Design review of the part shown in the three views and the two pictorial views. Dimensions are in mm from the part's minimum x, y and z. Give positions to 0.01 mm unless a question says otherwise; leave off trailing zeros. Order: outer loops, then holes, each group sorted by start corner. A loop starts at its lowest first (then second) coordinate and runs counter-clockwise, first axis right, second up. Notation, with made-up numbers: (-13, 73.25) - (20, 73.25) arc R17 cw to (20, 106.25) - close; hole circle Ø7 at (-23.5, 78). An arc over 180 degrees is marked (long way). Put each result on its own line as item: value.
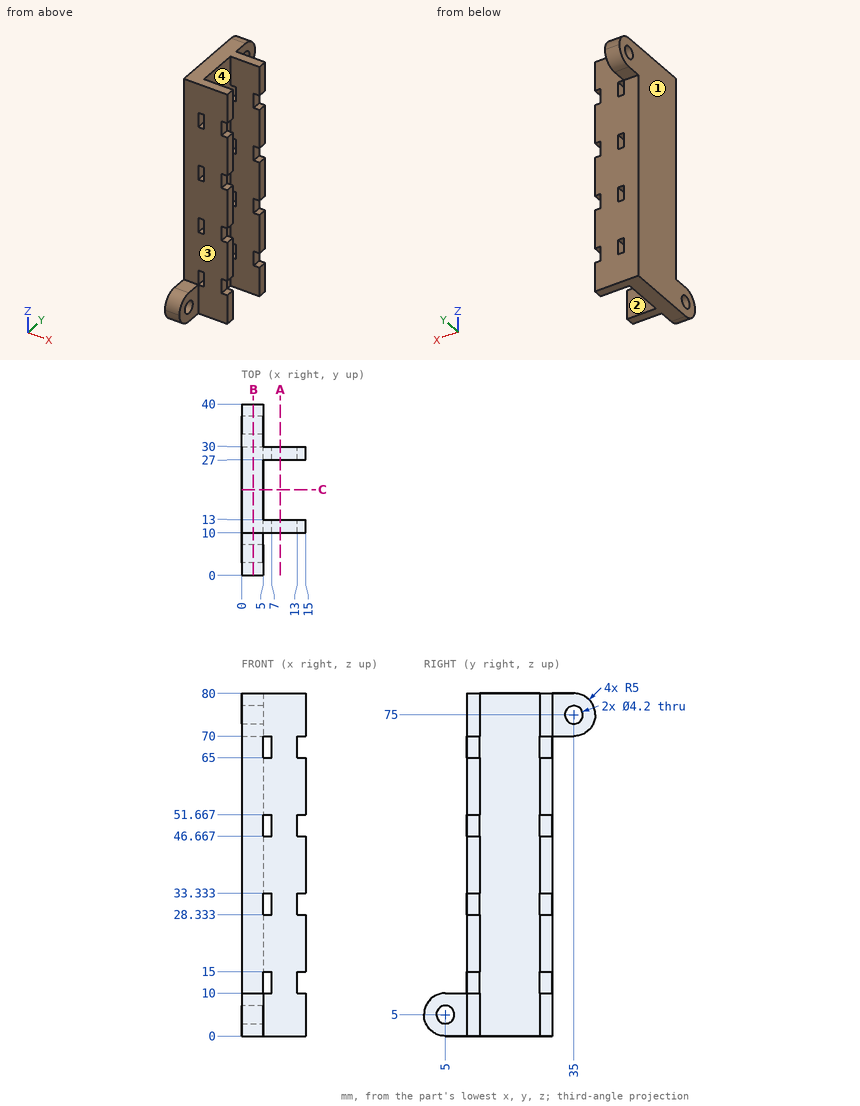
(1) Take a section at B-B, the plane x = 2.75. Count the separate pieces of the cut face and the enclosed holes in it, then the cut area to 3 significant figures.
The answers:
separate pieces: 1
enclosed holes: 2
area: 1,750 mm^2
(2) The part is to be moulded in two halves that separate along Y. For the marked faces 1, 2, 3 and 4, say which applies: pulls with the +Y half, pulls with the -Y half, needs draft (parallel to the pull), parting line crosses it, or undercut.
The answers:
face 1: needs draft
face 2: undercut
face 3: pulls with the -Y half
face 4: undercut
(3) Clearance check with flat-ended pins moving along their axes: pin 1 Ø1 at (x, y) = (14.5, 11.5) entering from -Z; pin 2 Ø5 at (x, z) = (3.5, 70.5) entering from -Y; pin 3 Ø2.5 at (y, z) = (12, 11.5) entering from +X; pin 4 Ø1 at (y, z) = (32, 49) entering from +X. State where each tip first meets the part, or that it passes through.
The answers:
pin 1: z = 0
pin 2: y = 10
pin 3: x = 13
pin 4: through
(4) Take a section at A-A, the plane x = 9. Write out the cut boundary in (y, z), then the cut area to 3 significant figures.
The answers:
outline: (10, 0) - (13, 0) - (13, 80) - (10, 80) - close; (27, 0) - (30, 0) - (30, 80) - (27, 80) - close
area: 480 mm^2
(5) Take a section at C-C, the plane y = 20. Write out the cut boundary in (x, z), then the cut area to 3 significant figures.
The answers:
outline: (0, 0) - (5, 0) - (5, 80) - (0, 80) - close
area: 400 mm^2
(6) Wall thickness on L1, parallel to Z at x = 14.25, y = 28.5; L2, parallel to Y at x = 2.2, z = 75; L3, parallel to Y at x = 6, z = 63.5: over which ranges is each line inside the solid? List them lowest first.
The answers:
L1: 0 to 10, 15 to 28.33, 33.33 to 46.67, 51.67 to 65, 70 to 80
L2: 10 to 32.9, 37.1 to 40
L3: 10 to 13, 27 to 30
